from build123d import *

# Parameters (mm, degrees)
SKETCH_1_R      = 6.5
SKETCH_1_R_2    = 1.5
EXTRUDE_1_DEPTH = 5
CHAMFER_1_SIZE  = 1
CHAMFER_2_SIZE  = 0.5


with BuildPart() as part:
    # 草图1 → 凸台-拉伸1 (new body)
    with BuildSketch(Plane.XY):
        Circle(SKETCH_1_R)
        Circle(SKETCH_1_R_2, mode=Mode.SUBTRACT)
    extrude(amount=EXTRUDE_1_DEPTH)

    # 倒角1
    chamfer_1_edges = [part.edges().sort_by_distance(p)[0] for p in [
        (-6.5, 0, 0),
        (-6.5, 0, 5),
    ]]
    chamfer(chamfer_1_edges, length=CHAMFER_1_SIZE)

    # 倒角2
    chamfer_2_edges = [part.edges().sort_by_distance(p)[0] for p in [
        (-1.5, 0, 0),
        (-1.5, 0, 5),
    ]]
    chamfer(chamfer_2_edges, length=CHAMFER_2_SIZE)


solid = part.part
Verification items for the finished model (mm, model axes). Coordinates: 2 decimals unless noted, no trailing zeros. Loops run counter-clockwise (first coordinate to the right, second up) from the corner with the lowest first, then second, coordinate; pieces in that order, holes last. Notation, with made-up numbers: (56, 48.25) -> (83, 48.25) arc R16 cw to (83, 69.25) -> close; hole circle Ø9 at (-21, 17.5). An arc over 180 degrees is marked (long way). Answer as CSV lines item,"result".
1) Cross-section at C-C, the plane z = 2.95. Record the cut outline in (x, y).
Found:
outline,"circle Ø13 at (0, 0); hole circle Ø3 at (0, 0)"
2) Depth check by flat-ended pin: pin 1 (1 mm diameter, centred on y = 1.5, z = 1.5, fed in from -X); pin 2 (3.5 mm diameter, centred on x = 0, y = 0, fed in from -Z). Enter the tip coordinate at first touch or a pass-through.
Found:
pin 1,"stops at x = -6.42"
pin 2,"stops at z = 0.25"
3) Cross-section at A-A, the plane x = 0. Record the cut outline in (y, z).
Found:
outline,"(-6.5, 1) -> (-5.5, 0) -> (-2, 0) -> (-1.5, 0.5) -> (-1.5, 4.5) -> (-2, 5) -> (-5.5, 5) -> (-6.5, 4) -> close; (1.5, 0.5) -> (2, 0) -> (5.5, 0) -> (6.5, 1) -> (6.5, 4) -> (5.5, 5) -> (2, 5) -> (1.5, 4.5) -> close"
4) Thickness scan on L1, parallel to Y at x = 0, z = 2; L2, parallel to Y at x = 1.25, z = 1.8; L3, parallel to X at y = -0.5, z = 4.05. Record the ranges inside material, lowest first. Write a range as from..to.
Found:
L1,"y = -6.5..-1.5, 1.5..6.5"
L2,"y = -6.38..-0.83, 0.83..6.38"
L3,"x = -6.43..-1.41, 1.41..6.43"
5) Release check for a two-part mould opening along Y. For faces 1 (the cylindrical face through (-1.5, 0.07, 2.47)), 2 (the cylindrical face through (-5.158, -3.955, 2.479)), 3 (the flat face through (-0.1, -2.4, 5)) record: +Y half, -Y half, draft (parallel to the pull), parting line (faces both ways), or undercut.
Found:
face 1,"undercut"
face 2,"parting line"
face 3,"draft"
